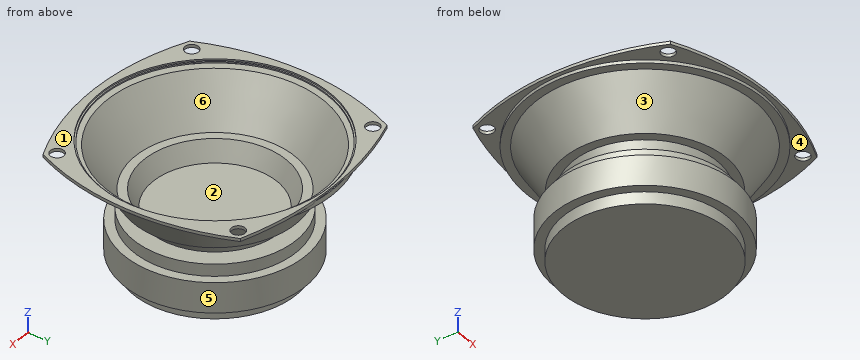
```python
from build123d import *

# Parameters (mm, degrees)
SKETCH001_R   = 2.25
SKETCH001_R_2 = 38.017291
PAD_DEPTH     = 1


with BuildPart() as part:
    # Sketch → Revolution (revolve)
    with BuildSketch(Plane.XZ):
        Polygon((0, 0), (27, 0), (27, 4), (30, 4), (30, 14), (27, 14), (27, 18), (21.287003, 18), (23.87335, 23.307098), (26.847654, 23.307098), (36.231567, 37.891254), (39.074654, 37.891254), (39, 39.5), (37.505909, 39.5), (37.505909, 39.066467), (38.493389, 39.066467), (38.493389, 38.34399), (35.97266, 38.34399), (26.419674, 23.90789), (23.58906, 23.90789), (20.568153, 17.960899), (0, 17.960899), align=None)
    revolve(axis=Axis((0, 0, 0), (0, 0, 1)))

    # Sketch001 → Pad (new body)
    with BuildSketch(Plane.XY.offset(39)):
        with BuildLine():
            ThreePointArc((33.120745, -33.120745), (40.25, 0), (33.120745, 33.120745))
            ThreePointArc((33.120745, 33.120745), (0, 38.620344), (-33.120745, 33.120745))
            ThreePointArc((-33.120745, 33.120745), (-40.25, 0), (-33.120745, -33.120745))
            ThreePointArc((-33.120745, -33.120745), (0, -40.397171), (33.120745, -33.120745))
        make_face()
        with Locations((-30.405592, 30.405592)):
            Circle(SKETCH001_R, mode=Mode.SUBTRACT)
        with Locations((30.405592, 30.405592)):
            Circle(SKETCH001_R, mode=Mode.SUBTRACT)
        with Locations((30.405592, -30.405592)):
            Circle(SKETCH001_R, mode=Mode.SUBTRACT)
        with Locations((-30.405592, -30.405592)):
            Circle(SKETCH001_R, mode=Mode.SUBTRACT)
        Circle(SKETCH001_R_2, mode=Mode.SUBTRACT)
    extrude(amount=PAD_DEPTH)


solid = part.part
```
The model under review builds one solid part; all positions refer to its coordinate system, in mm. Face numbers are marked on the shaded views. A direction names the side the tool comes from. Round coordinates to 2 decimals unless told otherwise and drop trailing zeros. Loops run counter-clockwise (first coordinate to the right, second up) from the corner with the lowest first, then second, coordinate; pieces in that order, holes last.
1) The part is to be moulded in two halves that separate along X. For the marked faces 4, 5 and 6, say which applies: pulls with the +X half, pulls with the -X half, needs draft (parallel to the pull), parting line crosses it, or undercut.
Values follow:
face 4: needs draft
face 5: parting line crosses it
face 6: undercut
2) Consider section A-A on z = 33. State the section outline as (x, y) points, then the cut area to 3 significant figures.
Values follow:
outline: circle Ø66.17 at (0, 0); hole circle Ø64.87 at (0, 0)
area: 133 mm2
3) Tool access review of the marked faces 1, 2 and 3: name each direction out of +Z, -Z, +X, -X, +Y, -Y from which nothing blocks a thin tool from reaching the whole face with its end or side.
Values follow:
face 1: +Z, +X, -X, +Y, -Y
face 2: +Z
face 3: none
4) Clearance check with flat-ended pins moving along their axes: P1, Ø12.5, axis at x = -7, y = 6, coming from the +Z side; P2, Ø1, axis at y = -24.5, z = 20.5, coming from the +X side; P3, Ø8, axis at x = -8, z = 14, coming from the +Y side; P4, Ø8, axis at y = 20.5, z = 7, coming from the +X side. State where each tip first meets the part, or that it passes through.
Values follow:
P1: stops at z = 17.96
P2: passes through
P3: stops at y = 29.73
P4: stops at x = 25.05
5) Wall thickness on line 1 along Z through (x, y) = (-16, -19); line 2 along X through (y, z) = (16, 20); line 3 along Y through (x, z) = (0, 39.3): over which ranges is each line inside the solid? List them lowest first.
Values follow:
line 1: z = 0 to 18, 23.31 to 23.91
line 2: x = -15.48 to -14.52, 14.52 to 15.48
line 3: y = -40.4 to -37.51, 37.51 to 39.01
